Check sheet for the modelled part. Datum: model origin and axes. Units: mm. A direction names the side the tool comes from. Round coordinates to 2 decimals unless told otherwise and drop trailing zeros. Write each loop counter-clockwise with the first axis right and the second up, starting at its lowest first coordinate (ties: lowest second). Pieces come first, ordered by that corner, then holes. Notation, with made-up numbers: (-14.75, -11) -> (38.25, -11) arc R16 ccw to (38.25, 9) -> close; hole circle Ø7 at (82.5, 7). An arc over 180 degrees is marked (long way). Write item = value, one per line.
from build123d import *

# Parameters (mm, degrees)
F2_SIZE  = 1
F3_SIZE  = 5
F5_W     = 154.381274
F5_H     = 110.501114
F6_DEPTH = 25


with BuildPart() as f1:
    # F0 (on Front) → F1 (revolve)
    with BuildSketch(Plane.XZ):
        Polygon((95, 10), (25, 10), (25, 0), (125, 0), (103.349365, 12.5), (100, 12.5), (100, 15), (95, 15), align=None)
    revolve(axis=Axis((75, 0, 0), (1, 0, 0)))

    # F2
    f2_edges = [f1.edges().sort_by_distance(p)[0] for p in [
        (100, 0, -15),
        (95, 0, -15),
    ]]
    chamfer(f2_edges, length=F2_SIZE)

    # F3
    f3_edges = [f1.edges().sort_by_distance(p)[0] for p in [
        (25, 0, -10),
    ]]
    chamfer(f3_edges, length=F3_SIZE)

    # F5 (on offset) → F6 (cut)
    with BuildSketch(Plane.XZ.offset(25)):
        with Locations((66.994385, 19.205375)):
            Rectangle(F5_W, F5_H)
    extrude(amount=-F6_DEPTH, mode=Mode.SUBTRACT)


solid = f1.part
(1) Sectioned sample at B-B on x = 53. Enter the section's corners in (y, z), then the cut area to 3 significant figures.
Worked answers:
outline = (0, -10) arc R10 ccw to (0, 10) -> close
area = 157 mm²
(2) Go/stop test with flat-tipped pins: P1, Ø6, axis at x = 68, z = 2, coming from the +Y side; P2, Ø1, axis at x = 43.5, y = 2.5, coming from the +Z side; P3, Ø3, axis at x = 46.5, y = 13, coming from the -Z side; P4, Ø3, axis at x = 81.5, z = -9, coming from the +Y side. Record where each tip stops, or that it passes through.
Worked answers:
P1 = 10
P2 = 9.8
P3 = through
P4 = 6.61
(3) Sectioned sample at A-A on z = 0. Enter the section's corners in (x, y), then the cut area to 3 significant figures.
Worked answers:
outline = (25, 0) -> (125, 0) -> (103.35, 12.5) -> (100, 12.5) -> (100, 14) -> (99, 15) -> (96, 15) -> (95, 14) -> (95, 10) -> (30, 10) -> (25, 5) -> close
area = 939 mm²
(4) Material ranges on L1, parallel to X at y = 3.25, z = 12.5; L2, parallel to Z at x = 101.5, y = 9.5; L3, parallel to X at y = 5.75, z = 5, recorded low to high. Write a range as [from, to].
Worked answers:
L1 = [95, 100]
L2 = [-8.12, 8.12]
L3 = [27.62, 111.8]
(5) Access from +Z, -Z, +X, -X, +Y, -Y to the whole of each face (thin tool, end or side, straight path). Record for faces 1 (the cylindrical face through (62, 10, 0)), 2 (the flat face through (25, 2, 0)), 3 (the cylindrical face through (101.651, 12.497, -0.275)).
Worked answers:
face_1 = -X, +Y
face_2 = +Z, -Z, -X, +Y, -Y
face_3 = +X, +Y
(6) Sectioned sample at C-C on x = 110. Enter the section's corners in (y, z), then the cut area to 3 significant figures.
Worked answers:
outline = (0, -8.66) arc R8.66 ccw to (0, 8.66) -> close
area = 118 mm²
